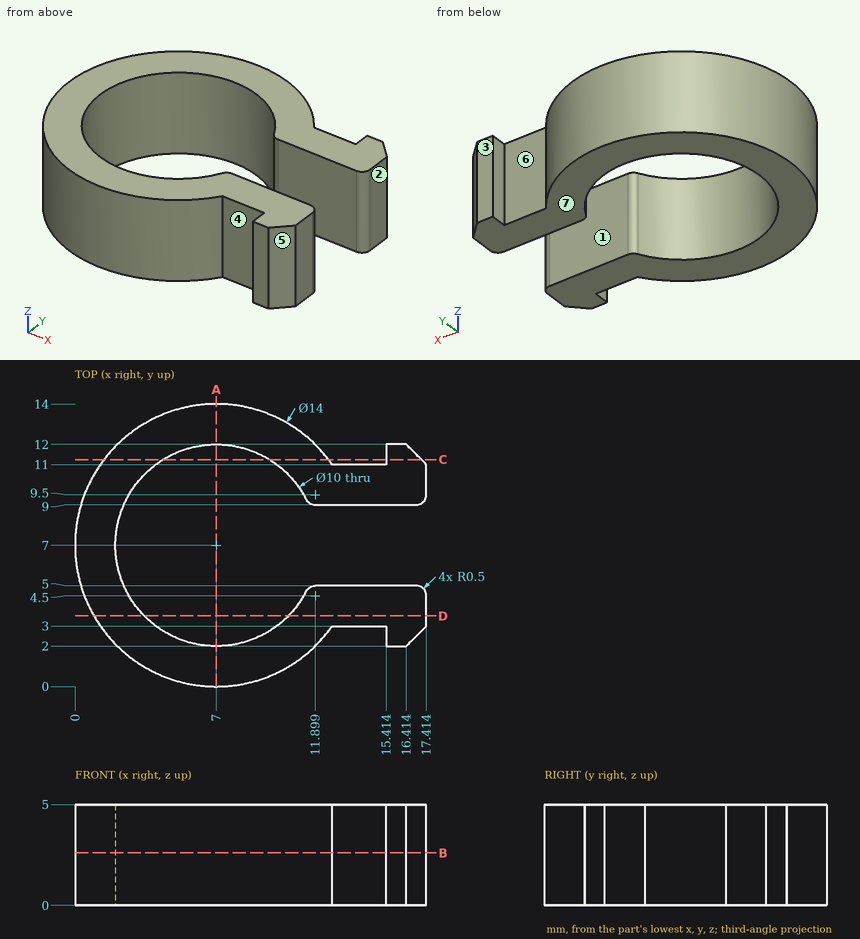
Design review of the part shown in the three views and the two pictorial views. Dimensions are in mm from the part's minimum x, y and z. A direction names the side the tool comes from. Give positions to 0.01 mm unless a question says otherwise; leave off trailing zeros. Loops run counter-clockwise (first coordinate to the right, second up) from the corner with the lowest first, then second, coordinate; pieces in that order, holes last. Notation, with made-up numbers: (23, 64) -> (61, 64) arc R11 ccw to (61, 81) -> close; hole circle Ø1 at (72.5, 36). An arc over 180 degrees is marked (long way). Answer as a JSON object with one key per item and string values. Group by question number.
Q1. Insertion check: pin 1 (0.5 mm diameter, centred on x = 16, z = 2.5, fed in from -Y); pin 2 (2 mm diameter, centred on y = 6.5, z = 0.5, fed in from +X); pin 3 (1.5 mm diameter, centred on x = 15, z = 2.5, fed in from +Y). Each pin has a flat end and moves straight along its axis. Give the tip position at first contact, or say it passes through.
Q2. Take a section at B-B (z = 2.6). Write out the cut boundary in (x, y), plus the area to 3 significant figures.
Q3. Tool access review of the marked faces 1, 2 and 3: name each direction out of +Z, -Z, +X, -X, +Y, -Y from which nothing blocks a thin tool from reaching the whole face with its end or side.
Q4. Take a section at D-D (y = 3.5). Write out the cut boundary in (x, z).
Q5. Take a section at C-C (y = 11.25). Write out the cut boundary in (x, z), plus the area to 3 significant figures.
Q6. Draft analysis for pull direction X (two halves, no side actions). For the marked faces 4, 5, 6 and 7, state which applies: pulls with the +X half, pulls with the -X half, needs draft (parallel to the pull), parting line crosses it, or undercut.
Q7. Wall thickness on line 1 along Y through (x, z) = (7, 3.4); line 2 along Y through (x, z) = (13.25, 0.25); line 3 along X through (y, z) = (11.5, 1.6) (1 decimal): over which ranges is each line inside the solid? List them lowest first.
Q8. Take a section at A-A (x = 7). Write out the cut boundary in (y, z), plus the area to 3 significant figures.
Answer below:
{
 "1": {"pin 1": "stops at y = 2", "pin 2": "stops at x = 2.23", "pin 3": "stops at y = 12"},
 "2": {"outline": "(11.45, 4.73) arc R5 cw (long way) to (11.45, 9.27) arc R0.5 ccw to (11.9, 9) -> (16.91, 9) arc R0.5 ccw to (17.41, 9.5) -> (17.41, 11) -> (16.41, 12) -> (15.41, 12) -> (15.41, 11) -> (12.74, 11) arc R7 ccw (long way) to (12.74, 3) -> (15.41, 3) -> (15.41, 2) -> (16.41, 2) -> (17.41, 3) -> (17.41, 4.5) arc R0.5 ccw to (16.91, 5) -> (11.9, 5) arc R0.5 ccw to start", "area": "86.6 mm2"},
 "3": {"face 1": "+Z, -Z, +X", "face 2": "+Z, -Z, +X, +Y, -Y", "face 3": "+Z, -Z, +X, +Y"},
 "4": {"outline": "(0.94, 0) -> (3.43, 0) -> (3.43, 5) -> (0.94, 5) -> close; (10.57, 0) -> (17.41, 0) -> (17.41, 5) -> (10.57, 5) -> close"},
 "5": {"outline": "(1.44, 0) -> (4.37, 0) -> (4.37, 5) -> (1.44, 5) -> close; (9.63, 0) -> (12.56, 0) -> (12.56, 5) -> (9.63, 5) -> close; (15.41, 0) -> (17.16, 0) -> (17.16, 5) -> (15.41, 5) -> close", "area": "38.0 mm2"},
 "6": {"face 4": "undercut", "face 5": "pulls with the +X half", "face 6": "undercut", "face 7": "needs draft"},
 "7": {"line 1": "y = 0 to 2, 12 to 14", "line 2": "y = 3 to 5, 9 to 11", "line 3": "x = 1.6 to 4.8, 9.2 to 12.4, 15.4 to 16.9"},
 "8": {"outline": "(0, 0) -> (2, 0) -> (2, 5) -> (0, 5) -> close; (12, 0) -> (14, 0) -> (14, 5) -> (12, 5) -> close", "area": "20.0 mm2"}
}
